Part model, mm, in its own coordinate system. Face numbers are marked on the shaded views. A direction names the side the tool comes from. Round coordinates to 2 decimals unless told otherwise and drop trailing zeros. Write each loop counter-clockwise with the first axis right and the second up, starting at its lowest first coordinate (ties: lowest second). Pieces come first, ordered by that corner, then holes. Notation, with made-up numbers: M 56.25,0.5 L 61.25,0.5 A15 ccw 61.25,18.5 Z; hole C 56.5,59 d1. An arc over 180 degrees is marked long. Use one line per item in the form item = value. Start each with the question number.
Item 1: Cut at A-A, the plane x = 0. Give the cut face in (y, z) (3 decimals), then the cut area to 3 significant figures.
Item 2: Flat gauge pins, fed straight in: pin 1 Ø3 at (x, z) = (-6, 7.5) entering from -Y; pin 2 Ø2 at (x, z) = (5, -1.5) entering from -Y. Where does each tip first touch, or does it go through?
Item 3: Mould opens along Z. For the marked faces 1, 2 and 3 say: +Z half, -Z half, draft (parallel to the pull), parting line (faces both ways), or undercut.
Item 4: Cut at B-B, the plane y = 5.75. Give the cut face in (x, z) (3 decimals), then the cut area to 3 significant figures.
Item 5: Cut at D-D, the plane z = -7. Give the cut face in (x, y).
Item 6: Probe L1, parallel to Z at x = 5.5, y = 5 (3 decimals); L2, parallel to Y at x = 4, z = -4.25; L3, parallel to Y at x = 0, z = 5.5. List the from-to ranges inside material, lowest first.
Item 7: Which spindle directions (+Z, -Z, +X, -X, +Y, -Y) get a long thin tool onto all of the face, cutting with end or side? Do the marked faces 4 and 5. Say none if no direction does.
Item 8: Cut at C-C, the plane y = 7.5. Give the cut face in (x, z) (3 decimals), then the cut area to 3 significant figures.
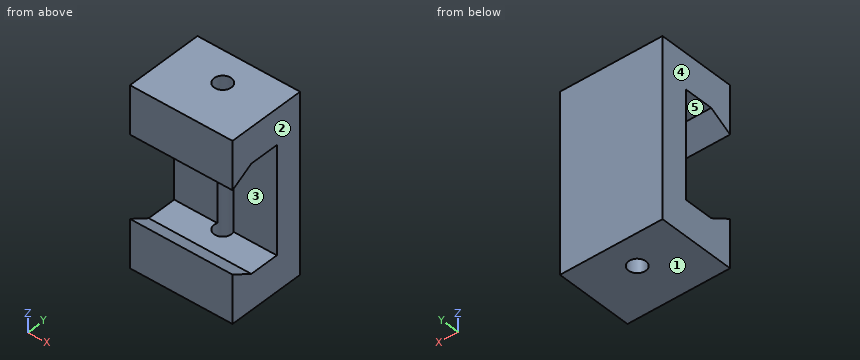
from build123d import *

# Parameters (mm, degrees)
BOSS_EXTRUDE1_DEPTH   = 8
F_6_32_TAPPED_HOLE1_D = 2.7051


with BuildPart() as part:
    # Sketch1 → Boss-Extrude1 (new, symmetric)
    with BuildSketch(Plane(origin=(0, 0, 0), x_dir=(0, 0, -1), z_dir=(1, 0, 0))):
        Polygon((-6.4, 0), (-8.375, 3.4), (-8.375, 8), (8.375, 8), (8.375, 3.4), (6.4, 0), (13.9, 0), (13.9, 12.2), (-13.9, 12.2), (-13.9, 0), align=None)
    extrude(amount=BOSS_EXTRUDE1_DEPTH, both=True)

    # #6-32 Tapped Hole1 (through all)
    with Locations(Plane.XY.offset(13.9)):
        with Locations((0, 7.5)):
            Hole(F_6_32_TAPPED_HOLE1_D / 2)


solid = part.part
Model answer:
q1.outline = M 0,-13.9 L 6.147,-13.9 L 6.147,-8.375 L 3.4,-8.375 L 0,-6.4 Z; M 0,6.4 L 3.4,8.375 L 6.147,8.375 L 6.147,13.9 L 0,13.9 Z; M 8.853,-13.9 L 12.2,-13.9 L 12.2,13.9 L 8.853,13.9 Z
q1.area = 168 mm²
q2.pin_1 = 0
q2.pin_2 = 8
q3.face_1 = -Z half
q3.face_2 = draft
q3.face_3 = undercut
q4.outline = M -8,-13.9 L 8,-13.9 L 8,-8.375 L -8,-8.375 Z; M -8,8.375 L 8,8.375 L 8,13.9 L -8,13.9 Z
q4.area = 177 mm²
q5.outline = M -8,0 L 8,0 L 8,1.03 L -8,1.03 Z; M -8,8 L -1.26,8 A1.35 cw 1.26,8 L 8,8 L 8,12.2 L -8,12.2 Z
q6.L1 = -13.9 to -8.375, 8.375 to 13.9
q6.L2 = 8 to 12.2
q6.L3 = 8.85 to 12.2
q7.face_4 = +Z, -Z, -X, +Y, -Y
q7.face_5 = +X, -X
q8.outline = M -8,-13.9 L -1.353,-13.9 L -1.353,-8.375 L -8,-8.375 Z; M -8,8.375 L -1.353,8.375 L -1.353,13.9 L -8,13.9 Z; M 1.353,-13.9 L 8,-13.9 L 8,-8.375 L 1.353,-8.375 Z; M 1.353,8.375 L 8,8.375 L 8,13.9 L 1.353,13.9 Z
q8.area = 147 mm²
